```python
from build123d import *

# Parameters (mm, degrees)
F1_DEPTH     = 76.2
F2_R         = 10.16
F3_DEPTH     = 76.2
F5_DEPTH     = 27.94
F7_DEPTH     = 15.24
F8_R         = 7.62
F9_DEPTH     = 10.16
F10_T1_DEPTH = 162.56
F11_T1_DEPTH = 162.56


# Not quite as in the source:
# - a fillet or chamfer that OpenCascade refuses, or shapes differently, is made with other operations: its cross-section is extruded or revolved along the edge and cut away or added


with BuildPart() as f1:
    # F0 (on Front) → F1 (new body)
    with BuildSketch(Plane.XZ):
        Polygon((0, 35.56), (0, 0), (111.76, 0), (147.32, 35.56), (147.32, 71.12), (111.76, 71.12), (76.2, 35.56), align=None)
    extrude(amount=F1_DEPTH)

    # F2 (on face) → F3 (cut)
    with BuildSketch(Plane.XZ.offset(76.2)):
        with Locations((93.98, 20.32)):
            Circle(F2_R)
    extrude(amount=-F3_DEPTH, mode=Mode.SUBTRACT)

    # F4 (on face) → F5 (cut)
    with BuildSketch(Plane.XY.offset(71.12)):
        with BuildLine():
            ThreePointArc((133.35, -15.24), (129.54, -11.43), (125.73, -15.24))
            Line((125.73, -15.24), (125.73, -60.96))
            ThreePointArc((125.73, -60.96), (129.54, -64.77), (133.35, -60.96))
            Line((133.35, -60.96), (133.35, -15.24))
        make_face()
    extrude(amount=-F5_DEPTH, mode=Mode.SUBTRACT)

    # F6 (on face) → F7 (cut)
    with BuildSketch(Plane.XY.offset(35.56)):
        with BuildLine():
            ThreePointArc((58.2606249903, -40.64), (58.3801171077, -39.3724975829), (58.42, -38.1))
            ThreePointArc((58.42, -38.1), (58.3801171077, -36.8275024171), (58.2606249903, -35.56))
            ThreePointArc((58.2606249903, -35.56), (38.1, -17.78), (17.9393750097, -35.56))
            ThreePointArc((17.9393750097, -35.56), (17.78, -38.1), (17.9393750097, -40.64))
            ThreePointArc((17.9393750097, -40.64), (38.1, -58.42), (58.2606249903, -40.64))
        make_face()
        with BuildLine():
            ThreePointArc((58.2606249903, -35.56), (58.3801171077, -36.8275024171), (58.42, -38.1))
            ThreePointArc((58.42, -38.1), (58.3801171077, -39.3724975829), (58.2606249903, -40.64))
            Line((58.2606249903, -40.64), (76.2, -40.64))
            Line((76.2, -40.64), (76.2, -35.56))
            Line((76.2, -35.56), (58.2606249903, -35.56))
        make_face()
        with BuildLine():
            ThreePointArc((17.9393750097, -40.64), (17.78, -38.1), (17.9393750097, -35.56))
            Line((17.9393750097, -35.56), (0, -35.56))
            Line((0, -35.56), (0, -40.64))
            Line((0, -40.64), (17.9393750097, -40.64))
        make_face()
    extrude(amount=-F7_DEPTH, mode=Mode.SUBTRACT)

    # F8 (on face) → F9 (cut)
    with BuildSketch(Plane.XY.offset(20.32)):
        with Locations((38.1, -38.1)):
            Circle(F8_R)
    extrude(amount=-F9_DEPTH, mode=Mode.SUBTRACT)

    # F10: fillet of radius 25.4 on 1 edges, made by hand

    # F10_s2 → F10_t1 (cut)
    with BuildSketch(Plane.XY.offset(-63.5)):
        with BuildLine():
            add(Edge.make_bspline(
                [(0, -50.8), (0, -76.2), (25.4, -76.2)],
                knots=[0, 0, 0, 1, 1, 1], degree=2, weights=[1, 4, 1]))
            Line((25.4, -76.2), (0, -76.2))
            Line((0, -76.2), (0, -50.8))
        make_face()
    extrude(amount=F10_T1_DEPTH, mode=Mode.SUBTRACT)

    # F11: fillet of radius 25.4 on 1 edges, made by hand

    # F11_s2 → F11_t1 (cut)
    with BuildSketch(Plane.XY.offset(-63.5)):
        with BuildLine():
            add(Edge.make_bspline(
                [(0, -25.4), (0, 0), (25.4, 0)],
                knots=[0, 0, 0, 1, 1, 1], degree=2, weights=[1, 4, 1]))
            Line((25.4, 0), (0, 0))
            Line((0, 0), (0, -25.4))
        make_face()
    extrude(amount=F11_T1_DEPTH, mode=Mode.SUBTRACT)


solid = f1.part
```
Model file for the job. Use its own axes, mm. A direction names the side the tool comes from. Coordinates: 2 decimals unless noted, no trailing zeros. Loops run counter-clockwise (first coordinate to the right, second up) from the corner with the lowest first, then second, coordinate; pieces in that order, holes last. Notation, with made-up numbers: (-38.75, -28) - (-21.75, -28) arc R19 cw to (-21.75, -5) - close; hole circle Ø9 at (28.25, 51). An arc over 180 degrees is marked (long way). Write item = value, one per line. Start each with the question number.
Item 1: 3-axis set-ups, long thin cutter, end or side, ignore diameter. For faces 4 (the face through (129, -38, 43.18)), 5 (the face through (39, -62, 35.56)), 6 (the face through (67, -40.64, 28)): which of +Z, -Z, +X, -X, +Y, -Y reach the whole face in a straight line?
Item 2: Pull direction Y, two halves, no side cores. Call faces 1 (the face through (85.917, -38.633, 14.138)), 2 (the face through (99, 0, 36)), 3 (the face through (125.73, -38, 57)): +Y half, -Y half, draft (parallel to the pull), parting line (faces both ways), or undercut.
Item 3: Saw through at B-B, the plane x = 38.1. List the corners of the cut face in (y, z), then the cut area to 3 significant figures.
Item 4: Saw through at C-C, the plane z = 45. List the corners of the cut face in (x, y).
Item 5: Wall check: probe 1 along X at (y, z) = (-20, 22); probe 2 along Z at (x, y) = (8, -10); probe 3 along Z at (x, y) = (93.98, -52.5). Give the ranges that are in metal, low to high. Write a range as [from, to].
Item 6: Saw through at D-D, the plane y = -43. List the corners of the cut face in (x, z).
Item 7: Saw through at A-A, the plane z = 56.5. List the corners of the cut face in (x, y).
Item 8: Drop flat-ended pins along their axis: pin 1 Ø8.5 at (y, z) = (-31.5, 51) entering from -X; pin 2 Ø2.5 at (x, y) = (128.5, -42.5) entering from +Z; pin 3 Ø10.5 at (x, y) = (27, -15.5) entering from +Z. Give the stop position or say it passes through.
Answers:
q1.face_4 = +Z
q1.face_5 = +Z, -X, +Y, -Y
q1.face_6 = +Z, -X
q2.face_1 = draft
q2.face_2 = +Y half
q2.face_3 = undercut
q3.outline = (-76.2, 0) - (0, 0) - (0, 35.56) - (-17.78, 35.56) - (-17.78, 20.32) - (-30.48, 20.32) - (-30.48, 10.16) - (-45.72, 10.16) - (-45.72, 20.32) - (-58.42, 20.32) - (-58.42, 35.56) - (-76.2, 35.56) - close
q3.area = 1,940 mm2
q4.outline = (85.64, -76.2) - (147.32, -76.2) - (147.32, 0) - (85.64, 0) - close; hole (125.73, -60.96) arc R3.81 ccw to (133.35, -60.96) - (133.35, -15.24) arc R3.81 ccw to (125.73, -15.24) - close
q5.probe_1 = [0.02, 28.86], [47.34, 83.96], [104, 133.76]
q5.probe_2 = [0, 35.56]
q5.probe_3 = [0, 10.16], [30.48, 53.34]
q6.outline = (0, 0) - (111.76, 0) - (147.32, 35.56) - (147.32, 71.12) - (133.35, 71.12) - (133.35, 43.18) - (125.73, 43.18) - (125.73, 71.12) - (111.76, 71.12) - (76.2, 35.56) - (57.82, 35.56) - (57.82, 20.32) - (43.94, 20.32) - (43.94, 10.16) - (32.26, 10.16) - (32.26, 20.32) - (18.38, 20.32) - (18.38, 35.56) - (0, 35.56) - close; hole circle Ø20.32 at (93.98, 20.32)
q7.outline = (97.14, -76.2) - (147.32, -76.2) - (147.32, 0) - (97.14, 0) - close; hole (125.73, -60.96) arc R3.81 ccw to (133.35, -60.96) - (133.35, -15.24) arc R3.81 ccw to (125.73, -15.24) - close
q8.pin_1 = 87.39
q8.pin_2 = 43.18
q8.pin_3 = 35.56
